Autodesk Inventor part; units mm, degrees
ref_plane "Work Plane1" through (-20, 0, 0) normal (1, 0, 0) x (0, 1, 0)
ref_plane "Work Plane2" through (0, 0, 0) normal (0, 0, 1) x (1, 0, 0)
ref_plane "Work Plane4" through (5.4558, -16.5513, 14.1595) normal (0.7071068, -0.7071068, 0) x (0, 0, -1)
sketch "Sketch1" plane through (0, 0, 0) normal (0, 0, 1) x (1, 0, 0)
  line L0 (15, 28.2088) -> (15.15, 10.0588)
  line L1 (13, 28.2088) -> (13.15, 10.0588)
  line L2 (13.15, 10.0588) -> (13.1595, 8.9045)
  line L3 (15.15, 10.0588) -> (15.1653, 8.2088)
  line L4 (15.1653, 8.2088) -> (10.25, -5.7912)
  line L5 (10.25, -5.7912) -> (10.25, -5.7912)
  line L6 (8, -5.7712) -> (8, -5.7912)
  line L7 (13.1595, 8.9045) -> (8, -5.7912)
  line L8 (15, 28.2088) -> (13, 28.2088)
  line L9 (0, -12.5912) -> (0, 35.0088) construction
  line L10 (-1, 0) -> (-1, 28.2088) construction
  line L11 (10.25, -5.7912) -> (8, -5.7912)
  line L12 (13.1595, 8.9045) -> (15.1595, 8.9045)
  point P0 (0, 0)
  point P1 (0, 0)
  point P2 (-1, 22.6667)
  dimension "d0" = 2
  dimension "d1" = 2
  dimension "d2" = 0
  dimension "d3" = 0
  dimension "d4" = 18.15
  dimension "d5" = 1.9999
  dimension "d6" = 14
  dimension "d7" = 0
  dimension "d8" = 1.85
  dimension "d9" = 2.123
  dimension "d10" = 1
revolve "Revolution1" add sketch "Sketch1" angle 360 about axis through (-1, 0, 0) along (0, 1, 0) contours L0 L3 L12 L2 L1 L8
ref_plane "Work Plane1" through (-20, 0, 0) normal (1, 0, 0) x (0, 1, 0)
sketch "Sketch2" plane through (-20, 0, 0) normal (1, 0, 0) x (0, 1, 0)
  line L0 (8.9045, 14.1595) -> (8.9045, -14.1595) construction
  line L1 (8.9045, 0) -> (-10.0955, 0) construction
  point P0 (0, 0)
  dimension "d13" = 19
sketch "Sketch3" plane through (-1, 8.9045, 0) normal (0, -1, 0) x (1, 0, 0)
  circle A0 centre (0, 0) radius 16.1595
  circle A1 centre (0, 0) radius 14.1595
  point P0 (1, 0)
revolve "Revolution2" add sketch "Sketch3" angle 90 about axis through (-20, 8.9045, 14.1595) along (0, 0, -1)
ref_plane "Work Plane2" through (0, 0, 0) normal (0, 0, 1) x (1, 0, 0)
sketch "Sketch4" plane through (0, 0, 0) normal (0, 0, 1) x (1, 0, 0)
  line L0 (-20, 6.0641) -> (-20, -26.255) construction
  line L1 (-20, -10.0955) -> (-35, -10.0955) construction
  line L2 (-35, -10.0955) -> (-55, -10.0955) construction
  line L3 (-55, -10.0955) -> (-55, 0.9045) construction
  line L4 (-35, -10.0955) -> (-35, 1.1545) construction
  line L5 (-35, 1.1545) -> (-55, 0.9045)
  line L6 (-55, 0.9045) -> (-55, -0.2955)
  line L7 (-55, -0.2955) -> (-35, -0.0455)
  line L8 (-20, -24.255) -> (-20, 4.0641)
  line L9 (-20, 4.0641) -> (-35, -0.0455)
  line L10 (-35, 1.1545) -> (-20, 6.0641)
  line L11 (-20, 6.0641) -> (-20, 4.0641)
  point P0 (0, 0)
  dimension "d16" = 15
  dimension "d17" = 20
  dimension "d18" = 11
  dimension "d19" = 11.25
  dimension "d20" = 1.2
  dimension "d21" = 1.2
revolve "Revolution3" add sketch "Sketch4" angle 360 about axis through (-35, -10.0955, 0) along (-1, 0, 0)
ref_plane "Work Plane4" through (5.4558, -16.5513, 14.1595) normal (0.7071068, -0.7071068, 0) x (0, 0, -1)
ref_plane "Work Plane3" through (-20, 8.9045, 14.1595) normal (0.7071068, -0.7071068, 0) x (0, 0, -1)
sketch "Sketch5" plane through (5.4558, -16.5513, 14.1595) normal (0.7071068, -0.7071068, 0) x (0, 0, -1)
  circle A0 centre (14.1595, 0.0528) radius 12.5
  point P0 (14.1595, 7.8457)
  dimension "d25" = 25
extrude "Extrusion1" add sketch "Sketch5" against normal up to surface
properties part number "Ambu90deg"
Could you check a few things on this model? Use its own coordinates, in mm. A direction names the side the tool comes from. Round coordinates to 2 decimals unless told otherwise and drop trailing zeros. Loops run counter-clockwise (first coordinate to the right, second up) from the corner with the lowest first, then second, coordinate; pieces in that order, holes last.
Q1. I want a section at A-A (y = 13). Write out the boundary of the cut face in (x, z), and give its area (3 significant figures).
Q2. On a 3-axis mill with a long thin cutter (end or side, diameter ignored), from which of +Z, -Z, +X, -X, +Y, -Y can I reach the whole of each face in a straight line? I mean faces 4 (the conical face through (-44.9, -5.5, -8.8)), 5 (the conical face through (-44.9, -18.9, -6.8)), 6 (the flat face through (-55, -20, 1)). Say none if no direction works.
Q3. Please list where these lines run through material, in increasing order: L1, parallel to X at y = 23, z = 5; L2, parallel to Y at x = -46, z = -7.5; L3, parallel to X at y = 23, z = 9.5.
Q4. For P1, Ø1, axis at x = 1.5, y = 6, coming from the -Z side; P2, Ø6, axis at x = -18, y = -14, coming from the -Z side; P3, Ø4, axis at x = -43, y = -16, coming from the -Z side, each with a flat end and sliding along its axis, tell me the tip position at first contact or that it passes through.
Q5. I want a section at B-B (x = -42.5). Write out the boundary of the cut face in (y, z), and give its area (3 significant figures).
Q6. Thinking about a two-plate mould opening in Y: for faces 1 (the flat face through (5.617, -16.39, 0.175)), 2 (the conical face through (-30.728, -21.305, 0.493)), 3 (the flat face through (-1.07, 28.209, 14.15)), which applies, pulls with the +Y half, pulls with the -Y half, needs draft (parallel to the pull), parting line crosses it, or undercut?
Answer below:
1. outline: circle Ø32.25 at (-1, 0); hole circle Ø28.25 at (-1, 0)
1. area: 190 mm2
2. face 4: none
2. face 5: -X
2. face 6: +Z, -Z, -X, +Y, -Y
3. L1: x = -16.24 to -14.12, 12.12 to 14.24
3. L2: y = -18.3 to -16.58, -3.61 to -1.9
3. L3: x = -13.93 to -11.34, 9.34 to 11.93
4. P1: stops at z = -16.01
4. P2: stops at z = -16.13
4. P3: stops at z = -10.44
5. outline: circle Ø22.31 at (-10.1, 0); hole circle Ø19.91 at (-10.1, 0)
5. area: 79.6 mm2
6. face 1: pulls with the -Y half
6. face 2: undercut
6. face 3: pulls with the +Y half
